The model under review builds one solid part; all positions refer to its coordinate system, in mm. A direction names the side the tool comes from. Round coordinates to 2 decimals unless told otherwise and drop trailing zeros. Loops run counter-clockwise (first coordinate to the right, second up) from the corner with the lowest first, then second, coordinate; pieces in that order, holes last. Notation, with made-up numbers: (-31.75, 2) -> (-19.75, 2) arc R18 cw to (-19.75, 18) -> close; hole circle Ø10 at (11, 71.25). An arc over 180 degrees is marked (long way). Write each question's results on one line, items separated by ' | '. Start each with the question number.
Item 1: We need section D-D (x = 7.25). Give the boundary of the cut face in (y, z).
Item 2: Mouldability with a two-part tool opening along X and no side actions: class faces 1 (the cylindrical face through (1.05, 8.96, 4.77)), 2 (the cylindrical face through (-3, 0, 3)), 3 (the flat face through (-1, -10, -1)), 4 (the flat face through (1, -10, 3.5)) as pulls with the +X half, pulls with the -X half, needs draft (parallel to the pull), parting line crosses it, or undercut.
Item 3: Clearance check with flat-ended pins moving along their axes: pin 1 Ø3 at (y, z) = (7.5, 4.5) entering from +X; pin 2 Ø2.5 at (x, y) = (0, -11.5) entering from +Z; pin 3 Ø2 at (x, y) = (15.5, -6) entering from +Z; pin 4 Ø1.5 at (x, y) = (2, 3) entering from -Z. State where each tip first meets the part, or that it passes through.
Item 4: For L1, parallel to Y at x = 0, z = 0.75; L2, parallel to Y at x = 0, z = 4.7; L3, parallel to X at y = 11.5, z = 1.7, list the stretches that pass through material, from the lowest coordinate up. Write a range as from..to.
Item 5: We need section B-B (y = -11.5). Give the boundary of the cut face in (x, z), and give its area (3 significant figures).
Item 6: Tool access review of faces 5 (the flat face through (16, 0, 6)), 6 (the flat face through (8.55, 19, 6)), 7 (the flat face through (11.06, 18.505, 1.693)), 8 (the flat face through (1, 13, 3.5)), 9 (the cylindrical face through (0.26, -9.517, -0.507)): name each direction out of +Z, -Z, +X, -X, +Y, -Y from which nothing blocks a thin tool from reaching the whole face with its end or side.
Item 7: We need section C-C (y = -0.5). Give the boundary of the cut face in (x, z), and give its area (3 significant figures).
from build123d import *

# Parameters (mm, degrees)
SKETCH1_R                       = 1.5
BOSS_EXTRUDE1_DEPTH             = 6
SKETCH2_R                       = 0.9
CUT_EXTRUDE1_DEPTH              = 35.146742158
BOSS_EXTRUDE2_START             = 7.9
SKETCH3_R                       = 0.9
BOSS_EXTRUDE2_DEPTH             = 7.9
CBORE_FOR_M2_5_SHCS1_AT_2_COUNT = 2
CBORE_FOR_M2_5_SHCS1_AT_2_PITCH = 23
CBORE_FOR_M2_5_SHCS1_AT_3_COUNT = 2
CBORE_FOR_M2_5_SHCS1_AT_3_PITCH = 23
BOSS_EXTRUDE3_START             = 1
SKETCH8_R                       = 2
SKETCH8_R_2                     = 1.5
BOSS_EXTRUDE3_DEPTH             = 1


with BuildPart() as part:
    # Sketch1 → Boss-Extrude1 (new body)
    with BuildSketch(Plane.XY):
        with BuildLine():
            Line((17, 14.5), (-8, 14.5))
            Line((-8, 14.5), (-8, 7.5))
            ThreePointArc((-8, 7.5), (-3, 0), (-8, -7.5))
            Line((-8, -7.5), (-8, -14.5))
            Line((-8, -14.5), (17, -14.5))
            Line((17, -14.5), (17, 14.5))
        make_face()
        with Locations((0, 11.5)):
            Circle(SKETCH1_R, mode=Mode.SUBTRACT)
        with Locations((0, -11.5)):
            Circle(SKETCH1_R, mode=Mode.SUBTRACT)
    extrude(amount=BOSS_EXTRUDE1_DEPTH)

    # Sketch2 → Cut-Extrude1 (cut, through all)
    with BuildSketch(Plane(origin=(0, 14.5, 0), x_dir=(1, 0, 0), z_dir=(0, 1, 0))):
        with Locations((13.5, -6)):
            Circle(SKETCH2_R)
    extrude(amount=-CUT_EXTRUDE1_DEPTH, mode=Mode.SUBTRACT)

    # Sketch3 → Boss-Extrude2 (add)
    with BuildSketch(Plane(origin=(0, 14.5, 0), x_dir=(1, 0, 0), z_dir=(0, 1, 0)).offset(BOSS_EXTRUDE2_START)):
        Polygon((13.5, -0.284232335), (8.55, -3.142116168), (8.55, -8.857883832), (13.5, -11.715767665), (18.45, -8.857883832), (18.45, -3.142116168), align=None)
        with Locations(Location((13.5, -6, 0), (0, 0, 270))):
            Circle(SKETCH3_R, mode=Mode.SUBTRACT)
    extrude(amount=-BOSS_EXTRUDE2_DEPTH)

    # Sketch6 → Cut-Revolve1 (revolve, cut)
    with BuildSketch(Plane(origin=(5.973076211, 0, 10.345671476), x_dir=(0.8660254037844388, 0, -0.49999999999999983), z_dir=(0.4999999999999998, 0, 0.8660254037844387)), mode=Mode.PRIVATE) as cut_revolve1_sk:
        with BuildLine():
            Line((9.591342951, 22.4), (9.591342951, 16.4))
            ThreePointArc((9.591342951, 16.4), (10.678390575, 19.807038489), (13.141342951, 22.4))
            Line((13.141342951, 22.4), (9.591342951, 22.4))
        make_face()
    revolve(cut_revolve1_sk.sketch.rotate(Axis((13.5, 22.4, 6), (0, -1, 0)), 210), axis=Axis((13.5, 22.4, 6), (0, -1, 0)), mode=Mode.SUBTRACT)

    # Sketch7 → CBORE for M2.5 SHCS1 (revolve, cut)
    with BuildSketch(Plane(origin=(0, -11.5, 6), x_dir=(0, -1, 0), z_dir=(1, 0, 0))):
        Polygon((0, 0), (0, 6), (1.45, 6), (1.45, 2.5), (2.75, 2.5), (2.75, 0), align=None)
    cbore_for_m2_5_shcs1 = revolve(axis=Axis((0, -11.5, 12.35), (0, 0, -1)), mode=Mode.SUBTRACT)

    # CBORE for M2.5 SHCS1 at 2: CBORE for M2.5 SHCS1 ×2
    with Locations(*[(0, i * CBORE_FOR_M2_5_SHCS1_AT_2_PITCH, 0) for i in range(1, CBORE_FOR_M2_5_SHCS1_AT_2_COUNT)]):
        add(cbore_for_m2_5_shcs1, mode=Mode.SUBTRACT)

    # CBORE for M2.5 SHCS1 at 3: CBORE for M2.5 SHCS1 ×2
    with Locations(*[(0, i * CBORE_FOR_M2_5_SHCS1_AT_3_PITCH, 0) for i in range(1, CBORE_FOR_M2_5_SHCS1_AT_3_COUNT)]):
        add(cbore_for_m2_5_shcs1, mode=Mode.SUBTRACT)

    # Sketch8 → Boss-Extrude3 (add)
    # profile 1 of 2: a face of its own
    with BuildSketch(Plane(origin=(0, 0, 0), x_dir=(-1, 0, 0), z_dir=(0, 0, -1)).offset(BOSS_EXTRUDE3_START)):
        with Locations((0, 11.5)):
            Circle(SKETCH8_R)
        with Locations((0, 11.5)):
            Circle(SKETCH8_R_2, mode=Mode.SUBTRACT)
    # profile 2 of 2: a face of its own
    with BuildSketch(Plane(origin=(0, 0, 0), x_dir=(-1, 0, 0), z_dir=(0, 0, -1)).offset(BOSS_EXTRUDE3_START)):
        with Locations((0, -11.5)):
            Circle(SKETCH8_R)
        with Locations((0, -11.5)):
            Circle(SKETCH8_R_2, mode=Mode.SUBTRACT)
    extrude(amount=-BOSS_EXTRUDE3_DEPTH)


solid = part.part
Here are the results:
1) outline: (-14.5, 0) -> (14.5, 0) -> (14.5, 6) -> (-14.5, 6) -> close
2) face 1: undercut | face 2: pulls with the -X half | face 3: needs draft | face 4: undercut
3) pin 1: stops at x = 17 | pin 2: passes through | pin 3: stops at z = 6 | pin 4: stops at z = 0
4) L1: y = -14.5..-13, -10..10, 13..14.5 | L2: y = -14.5..-14.25, -8.75..8.75, 14.25..14.5 | L3: x = -8..-1.5, 1.5..17
5) outline: (-8, 0) -> (-2, 0) -> (-2, -1) -> (-1.5, -1) -> (-1.5, 3.5) -> (-2.75, 3.5) -> (-2.75, 6) -> (-8, 6) -> close; (1.5, -1) -> (2, -1) -> (2, 0) -> (17, 0) -> (17, 6) -> (14.4, 6) arc R0.9 cw to (12.6, 6) -> (2.75, 6) -> (2.75, 3.5) -> (1.5, 3.5) -> close | area: 125 mm2
6) face 5: +Z, +X, -X, -Y | face 6: +Z, -Z, -X, +Y | face 7: -Z, -X, +Y | face 8: +Z | face 9: -Z
7) outline: (-3.02, 0) -> (17, 0) -> (17, 6) -> (14.4, 6) arc R0.9 cw to (12.6, 6) -> (-3.02, 6) -> close | area: 119 mm2
